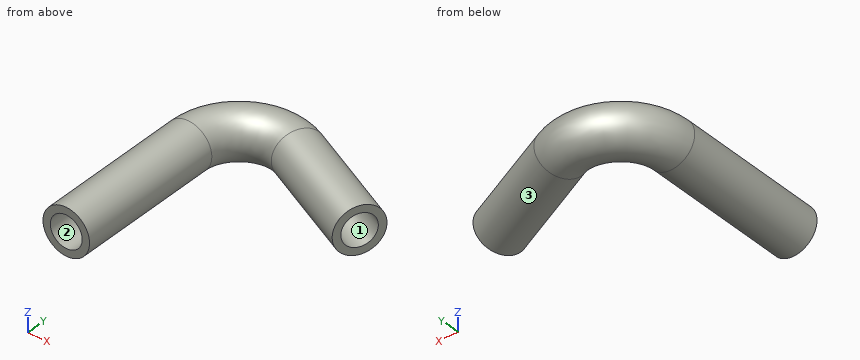
```python
from build123d import *

# Parameters (mm, degrees)
SWEEP_SOTTILE1_PROFILE_R   = 3.175
SWEEP_SOTTILE1_PROFILE_R_2 = 2.175


with BuildPart() as part:
    # Sweep-Sottile1: sweep along a path in Schizzo1
    with BuildLine(Plane.XY) as sweep_sottile1_path:
        Line((0, 0), (0, 20))
        ThreePointArc((0, 20), (3.189533949, 25.813752694), (9.80653858, 26.247454091))
        Line((9.80653858, 26.247454091), (23.401155386, 19.908180165))
    # Sweep-Sottile1 profile (on start of the path) → Sweep-Sottile1 (sweep)
    with BuildSketch(Plane.ZX):
        Circle(SWEEP_SOTTILE1_PROFILE_R)
        Circle(SWEEP_SOTTILE1_PROFILE_R_2, mode=Mode.SUBTRACT)
    sweep(path=sweep_sottile1_path.line)


solid = part.part
```
The model under review builds one solid part; all positions refer to its coordinate system, in mm. Face numbers are marked on the shaded views. Round coordinates to 2 decimals unless told otherwise and drop trailing zeros. Order: outer loops, then holes, each group sorted by start corner. A loop starts at its lowest first (then second) coordinate and runs counter-clockwise, first axis right, second up.
(1) Take a section at C-C, the plane z = -1.75. State the section outline as (x, y) points.
Working result:
outline: (-2.65, 0) - (-1.29, 0) - (-1.29, 20) arc R8.18 cw to (10.35, 27.42) - (23.95, 21.08) - (24.52, 22.31) - (10.93, 28.65) arc R9.54 ccw to (-2.65, 20) - close; (1.29, 0) - (2.65, 0) - (2.65, 20) arc R4.24 cw to (8.69, 23.85) - (22.28, 17.51) - (22.86, 18.74) - (9.26, 25.08) arc R5.6 ccw to (1.29, 20) - close
(2) Take a section at B-B, the plane y = 6. State the section outline as (x, z) points (3 decimals).
Working result:
outline: circle Ø6.35 at (0, 0); hole circle Ø4.35 at (0, 0)
(3) For P1, Ø1.5, axis at x = 12, z = 1.5, coming from the +Y side; P2, Ø1, axis at y = 11.5, z = -2, coming from the -X side; P3, Ø3, axis at x = 8.5, z = 0.5, coming from the -Y side, all flat-tipped, find the tip position at first contact; note any pin that passes through.
Working result:
P1: stops at y = 28.81
P2: stops at x = -2.8
P3: stops at y = 22.67
(4) Mouldability with a two-part tool opening along Z and no side actions: class the marked faces 1, 2 and 3 as released by +Z, released by -Z, zero draft, split by the parting line, or undercut.
Working result:
face 1: undercut
face 2: undercut
face 3: split by the parting line
(5) Wall thickness on L1, parallel to X at y = 5.75, z = 0 (3 decimals); L2, parallel to X at y = 20, z = -0.5; L3, parallel to Y at x = 15.75, z = -0.75: over which ranges is each line inside the solid? List them lowest first.
Working result:
L1: x = -3.175 to -2.175, 2.175 to 3.175
L2: x = -3.14 to -2.12, 2.12 to 3.14, 15.79 to 18.2
L3: y = 20.07 to 21.22, 25.73 to 26.88
(6) Take a section at A-A, the plane z = 0. State the section outline as (x, y) points (3 decimals).
Working result:
outline: (-3.175, 0) - (-2.175, 0) - (-2.175, 20) arc R9.068 cw to (10.726, 28.219) - (24.32, 21.879) - (24.743, 22.786) - (11.148, 29.125) arc R10.068 ccw to (-3.175, 20) - close; (2.175, 0) - (3.175, 0) - (3.175, 20) arc R3.718 cw to (8.465, 23.37) - (22.059, 17.031) - (22.482, 17.937) - (8.887, 24.276) arc R4.718 ccw to (2.175, 20) - close
